from build123d import *

# Parameters (mm, degrees)
F0_W     = 17.000006
F0_H     = 34.925
F0_W_2   = 17
F1_DEPTH = 25


with BuildPart() as f1:
    # F0 (on Top) → F1 (new body)
    with BuildSketch(Plane.XY):
        Polygon((54.175042, -81.352925), (54.175042, 45.647371), (-85.824958, 45.647357), (-85.824958, -81.352925), align=None)
        with Locations((-73.324955, -59.890378)):
            Rectangle(F0_W, F0_H, mode=Mode.SUBTRACT)
        Polygon((-49.584462, -77.352878), (-60.824958, -77.586921), (-60.824958, -49.586921), (-18.324958, -49.586921), (-18.324958, -61.310325), (-18.324958, -77.352878), align=None, mode=Mode.SUBTRACT)
        Polygon((29.175042, -49.586921), (29.175042, -77.586921), (17.934547, -77.352878), (-13.324958, -77.352878), (-13.324958, -61.310325), (-13.324958, -49.586921), align=None, mode=Mode.SUBTRACT)
        with Locations((41.675042, -60.124421)):
            Rectangle(F0_W_2, F0_H, mode=Mode.SUBTRACT)
        Polygon((29.175042, 9.881367), (29.175042, -10.852675), (29.175042, -24.852878), (29.175042, -45.586921), (-13.324958, -45.586921), (-13.324958, -19.852878), (-13.324958, -15.852675), (-13.324958, 9.881367), align=None, mode=Mode.SUBTRACT)
        Polygon((50.175042, 2.722325), (50.175042, -10.852675), (50.175042, -24.852878), (50.175042, -38.661921), (33.175042, -38.661921), (33.175042, -24.852878), (33.175042, -10.852675), (33.175042, 2.722325), align=None, mode=Mode.SUBTRACT)
        Polygon((-64.824954, 2.722325), (-64.824952, -10.852675), (-64.824952, -24.852878), (-64.824952, -38.427878), (-81.824958, -38.427878), (-81.824958, -24.852878), (-81.824958, -10.852675), (-81.824958, 2.722325), align=None, mode=Mode.SUBTRACT)
        Polygon((-18.324958, 9.881367), (-18.324958, -15.852675), (-18.324958, -19.852878), (-18.324958, -45.586921), (-60.824958, -45.586921), (-60.824958, -24.852878), (-60.824958, -10.852675), (-60.824954, 9.881367), align=None, mode=Mode.SUBTRACT)
        Polygon((-81.824958, 6.722325), (-81.824958, 41.647325), (-64.824957, 41.647325), (-64.824954, 6.722325), align=None, mode=Mode.SUBTRACT)
        Polygon((-60.824955, 13.881367), (-60.824958, 41.881367), (-49.584462, 41.647325), (-18.324958, 41.647325), (-18.324958, 25.604771), (-18.324958, 13.881367), align=None, mode=Mode.SUBTRACT)
        Polygon((17.934547, 41.647325), (29.175042, 41.881367), (29.175042, 13.881367), (-13.324958, 13.881367), (-13.324958, 25.604771), (-13.324958, 41.647325), align=None, mode=Mode.SUBTRACT)
        with Locations((41.675042, 24.184825)):
            Rectangle(F0_W_2, F0_H, mode=Mode.SUBTRACT)
    extrude(amount=F1_DEPTH)


solid = f1.part
Model file for the job. Use its own axes, mm. Round coordinates to 2 decimals unless told otherwise and drop trailing zeros. Loops run counter-clockwise (first coordinate to the right, second up) from the corner with the lowest first, then second, coordinate; pieces in that order, holes last. Notation, with made-up numbers: (40, 6) - (79, 6) arc R15 cw to (79, 12) - close; hole circle Ø1 at (-13.75, -19). An arc over 180 degrees is marked (long way). Write each question's results on one line, items separated by ' | '.
(1) Saw through at B-B, the plane x = 41. List the corners of the cut face in (y, z), then the cut area to 3 significant figures.
Answer below:
outline: (-81.35, 0) - (-77.59, 0) - (-77.59, 25) - (-81.35, 25) - close; (-42.66, 0) - (-38.66, 0) - (-38.66, 25) - (-42.66, 25) - close; (2.72, 0) - (6.72, 0) - (6.72, 25) - (2.72, 25) - close; (41.65, 0) - (45.65, 0) - (45.65, 25) - (41.65, 25) - close | area: 394 mm^2
(2) Saw through at C-C, the plane y = -32.5. List the corners of the cut face in (x, z), then the cut area to 3 significant figures.
Answer below:
outline: (-85.82, 0) - (-81.82, 0) - (-81.82, 25) - (-85.82, 25) - close; (-64.82, 0) - (-60.82, 0) - (-60.82, 25) - (-64.82, 25) - close; (-18.32, 0) - (-13.32, 0) - (-13.32, 25) - (-18.32, 25) - close; (29.18, 0) - (33.18, 0) - (33.18, 25) - (29.18, 25) - close; (50.18, 0) - (54.18, 0) - (54.18, 25) - (50.18, 25) - close | area: 525 mm^2
(3) Saw through at A-A, the plane y = -48. List the corners of the cut face in (x, z), then the cut area to 3 significant figures.
Answer below:
outline: (-85.82, 0) - (-81.82, 0) - (-81.82, 25) - (-85.82, 25) - close; (-64.82, 0) - (33.18, 0) - (33.18, 25) - (-64.82, 25) - close; (50.18, 0) - (54.18, 0) - (54.18, 25) - (50.18, 25) - close | area: 2,650 mm^2
(4) Wall check: L1, parallel to Y at x = -75, z = 15.5; L2, parallel to X at y = -75.5, z = 17.25; L3, parallel to Y at x = -12.5, z = 23. Give the ranges that are in metal, low to high.
Answer below:
L1: y = -81.35 to -77.35, -42.43 to -38.43, 2.72 to 6.72, 41.65 to 45.65 | L2: x = -85.82 to -81.82, -64.82 to -60.82, -18.32 to -13.32, 29.18 to 33.18, 50.18 to 54.18 | L3: y = -81.35 to -77.35, -49.59 to -45.59, 9.88 to 13.88, 41.65 to 45.65
(5) Mould opens along Y. For faces 1 (the flat face through (54.175, -19, 12)), 2 (the flat face through (-73, 2.722, 12)), 3 (the flat face through (-15, 45.647, 12)), 4 (the flat face through (42, 2.722, 12)) say: released by +Y, released by -Y, zero draft, split by the parting line, or undercut.
Answer below:
face 1: zero draft | face 2: undercut | face 3: released by +Y | face 4: undercut
(6) Saw through at D-D, the plane x = -72. List the corners of the cut face in (y, z).
Answer below:
outline: (-81.35, 0) - (-77.35, 0) - (-77.35, 25) - (-81.35, 25) - close; (-42.43, 0) - (-38.43, 0) - (-38.43, 25) - (-42.43, 25) - close; (2.72, 0) - (6.72, 0) - (6.72, 25) - (2.72, 25) - close; (41.65, 0) - (45.65, 0) - (45.65, 25) - (41.65, 25) - close
